```python
from build123d import *

# Parameters (mm, degrees)
F1_DEPTH = 2.5
F2_DEPTH = 2.5
F3_SIZE  = 2.49999


# Not quite as in the source:
# - a fillet or chamfer is up to 0.001 mm smaller than in the source, because OpenCascade refuses the exact size
# - a feature names something its author has since deleted; it is built from what else it names


with BuildPart() as f1:
    # F0 (on Top) → F1 (new body)
    with BuildSketch(Plane.XY):
        with BuildLine():
            ThreePointArc((-26.0619375711, 16.0619375711), (-20.9738946132, 0.5595870881), (-6.0619375711, -6.0619375711))
            Line((-6.0619375711, -6.0619375711), (-6.0619375711, 6.0619375711))
            ThreePointArc((-6.0619375711, 6.0619375711), (-17.2422774586, 8.7012577961), (-26.0619375711, 16.0619375711))
        make_face()
    extrude(amount=F1_DEPTH)

    # F0 (on Top) → F2 (join)
    with BuildSketch(Plane.XY):
        with BuildLine():
            Line((-6.0619375711, 6.0619375711), (-6.0619375711, -6.0619375711))
            ThreePointArc((-6.0619375711, -6.0619375711), (5.1184023164, -8.7012577961), (13.9380624289, -16.0619375711))
            ThreePointArc((13.9380624289, -16.0619375711), (8.8500194711, -0.5595870881), (-6.0619375711, 6.0619375711))
        make_face()
    extrude(amount=F2_DEPTH)

    # F3 (size 2.5 in the source; OpenCascade refuses exactly that, so slightly less here)
    f3_edges = [f1.edges().sort_by_distance(p)[0] for p in [
        (-20.973895, 0.559587, 2.5),
        (8.850019, -0.559587, 2.5),
    ]]
    chamfer(f3_edges, length=F3_SIZE)


solid = f1.part
```
Geometry: final body of the model. Coordinates: model frame, mm. Coordinates: 2 decimals unless noted, no trailing zeros. Order: outer loops, then holes, each group sorted by start corner. A loop starts at its lowest first (then second) coordinate and runs counter-clockwise, first axis right, second up. Notation, with made-up numbers: M 38,33 L 43,33 A24 ccw 43,43 Z; hole C 49.25,18.5 d4. An arc over 180 degrees is marked long. Answer in a Markdown table with one row per item. Add a question column.
Q1. Section query A-A on z = 1.1. Return the cut outline in (x, y), and give its area (3 significant figures).
Q2. Line query: L1, parallel to X at y = 8.5, z = 1; L2, parallel to X at y = 1, z = 0.7; L3, parallel to Z at x = 6, y = -7.5. Output: solid intervals per line, ascending.
Q3. Mould query, pull axis Z, two halves, no side actions, for faces 1 (the flat face through (-6, -1, 0)), 2 (the flat face through (-6, 1, 2.5)). Classes: released by +Z, released by -Z, zero draft, split by the parting line, or undercut.
Q4. Contact query for a flat-ended pin moving along its axis: P1, Ø10, axis at x = -21, y = -6, coming from the +Z side. Output: stop coordinate, or through.
Completed:
| question | item | result |
|---|---|---|
| 1 | outline | M -25.04,13.15 A19 ccw -6.06,-4.96 A26.1 cw 12.92,-13.15 A19 ccw -6.06,4.96 A26.1 cw Z |
| 1 | area | 319 mm2 |
| 2 | L1 | x = -24.34 to -18.98 |
| 2 | L2 | x = -20.43 to 6.2 |
| 2 | L3 | z = 0 to 1.47 |
| 3 | face 1 | released by -Z |
| 3 | face 2 | released by +Z |
| 4 | P1 | stops at z = 0.11 |
